```python
from build123d import *

# Parameters (mm, degrees)
F0_W     = 101.6
F0_H     = 101.6
F0_R     = 3.175
F0_R_2   = 4.7625
F0_R_3   = 12.7
F1_DEPTH = 9.525
F3_DEPTH = 3.81


with BuildPart() as f1:
    # F0 (on Top) → F1 (new body)
    with BuildSketch(Plane.XY):
        with Locations((50.8, 50.8)):
            Rectangle(F0_W, F0_H)
        with Locations((12.7, 12.7)):
            Circle(F0_R, mode=Mode.SUBTRACT)
        with Locations((23.859232, 23.859232)):
            Circle(F0_R_2, mode=Mode.SUBTRACT)
        with Locations((50.8, 50.8)):
            Circle(F0_R_3, mode=Mode.SUBTRACT)
        with Locations((77.740768, 23.859232)):
            Circle(F0_R_2, mode=Mode.SUBTRACT)
        with Locations((88.9, 12.7)):
            Circle(F0_R, mode=Mode.SUBTRACT)
        with Locations((23.859232, 77.740768)):
            Circle(F0_R_2, mode=Mode.SUBTRACT)
        with Locations((12.7, 88.9)):
            Circle(F0_R, mode=Mode.SUBTRACT)
        with Locations((77.740768, 77.740768)):
            Circle(F0_R_2, mode=Mode.SUBTRACT)
        with Locations((88.9, 88.9)):
            Circle(F0_R, mode=Mode.SUBTRACT)
    extrude(amount=F1_DEPTH)

    # F2 (on face) → F3 (cut)
    with BuildSketch(Plane.XY.offset(9.525)):
        with BuildLine():
            Line((6.35, 25.4), (6.35, 76.2))
            ThreePointArc((6.35, 76.2), (4.490128, 80.690128), (0, 82.55))
            Line((0, 82.55), (0, 19.05))
            ThreePointArc((0, 19.05), (4.490128, 20.909872), (6.35, 25.4))
        make_face()
        with BuildLine():
            Line((101.6, 19.05), (101.6, 82.55))
            ThreePointArc((101.6, 82.55), (97.109872, 80.690128), (95.25, 76.2))
            Line((95.25, 76.2), (95.25, 25.4))
            ThreePointArc((95.25, 25.4), (97.109872, 20.909872), (101.6, 19.05))
        make_face()
    extrude(amount=-F3_DEPTH, mode=Mode.SUBTRACT)


solid = f1.part
```
Verification items for the finished model (mm, model axes). A direction names the side the tool comes from. Round coordinates to 2 decimals unless told otherwise and drop trailing zeros. Order: outer loops, then holes, each group sorted by start corner. A loop starts at its lowest first (then second) coordinate and runs counter-clockwise, first axis right, second up. Notation, with made-up numbers: (60, 73.5) -> (70, 73.5) arc R8 ccw to (70, 88.5) -> close; hole circle Ø9 at (73, 79.5). An arc over 180 degrees is marked (long way). Put each result on its own line as item: value. Start each with the question number.
(1) Draft check along X on faces 1 (the face through (82.14, 75.92, 4.7)), 2 (the face through (97.16, 80.74, 7.65)), 3 (the face through (4.54, 80.64, 7.65)). Enter one of: +X half, -X half, draft (parallel to the pull), parting line (faces both ways), or undercut.
(2) Section check B-B (y = 50.8). Enter the section's corners in (x, z) (3 decimals).
(3) Material ranges on line 1 along Y through (x, z) = (89, 1.5); line 2 along Y through (x, z) = (77.5, 8), recorded low to high.
(4) Depth check by flat-ended pin: pin 1 Ø11 at (x, y) = (77.74, 77.74) entering from +Z (3 decimals); pin 2 Ø7 at (x, y) = (2.5, 44) entering from +Z (3 decimals). Enter the tip coordinate at first touch or a pass-through.
(5) Section check C-C (x = 50.8). Enter the section's corners in (y, z) (3 decimals), then the cut area to 3 significant figures.
(6) Section check A-A (x = 88.9). Enter the section's corners in (y, z) (3 decimals).
(7) Tool access check on faces 4 (the face through (0, 50, 4)), 5 (the face through (4.44, 20.86, 7.65)), 6 (the face through (97.06, 20.96, 7.65)). Record the directions out of +Z, -Z, +X, -X, +Y, -Y that give a thin tool (end or side, any length) a straight path to the whole face; none if there is none.
Completed:
1. face 1: undercut
1. face 2: +X half
1. face 3: -X half
2. outline: (0, 0) -> (38.1, 0) -> (38.1, 9.525) -> (6.35, 9.525) -> (6.35, 5.715) -> (0, 5.715) -> close; (63.5, 0) -> (101.6, 0) -> (101.6, 5.715) -> (95.25, 5.715) -> (95.25, 9.525) -> (63.5, 9.525) -> close
3. line 1: y = 0 to 9.53, 15.87 to 85.73, 92.07 to 101.6
3. line 2: y = 0 to 19.1, 28.62 to 72.98, 82.5 to 101.6
4. pin 1: stops at z = 9.525
4. pin 2: stops at z = 5.715
5. outline: (0, 0) -> (38.1, 0) -> (38.1, 9.525) -> (0, 9.525) -> close; (63.5, 0) -> (101.6, 0) -> (101.6, 9.525) -> (63.5, 9.525) -> close
5. area: 726 mm2
6. outline: (0, 0) -> (9.525, 0) -> (9.525, 9.525) -> (0, 9.525) -> close; (15.875, 0) -> (85.725, 0) -> (85.725, 9.525) -> (15.875, 9.525) -> close; (92.075, 0) -> (101.6, 0) -> (101.6, 9.525) -> (92.075, 9.525) -> close
7. face 4: +Z, -Z, -X, +Y, -Y
7. face 5: +Z, -X
7. face 6: +Z, +X
